Work out the finished part from the listing and answer in its coordinate system (mm). Face numbers are marked on the shaded views. A direction names the side the tool comes from. Give positions to 0.01 mm unless a question says otherwise; leave off trailing zeros. Loops run counter-clockwise (first coordinate to the right, second up) from the corner with the lowest first, then second, coordinate; pieces in that order, holes last. Notation, with made-up numbers: (-39, -4) - (-4, -4) arc R16 cw to (-4, 13) - close; hole circle Ø3 at (61, -2). An arc over 180 degrees is marked (long way). One line per item, written item: value.
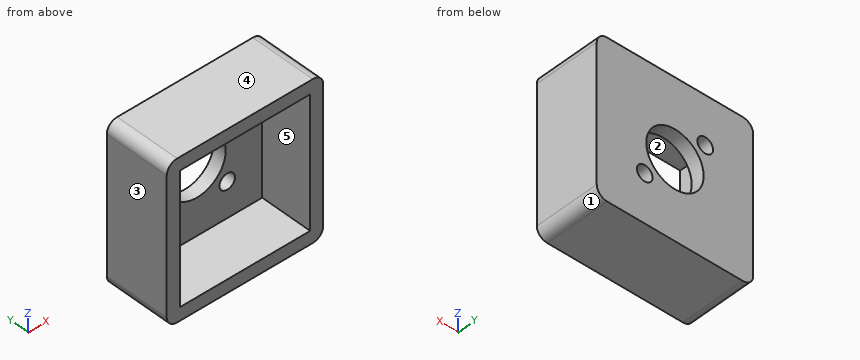
from build123d import *

# Parameters (mm, degrees)
SKETCH1_W           = 38.1
SKETCH1_H           = 38.1
SKETCH1_R           = 1.905
SKETCH1_R_2         = 6.985
BOSS_EXTRUDE1_DEPTH = 3.175
SKETCH1_3_W         = 38.1
SKETCH1_3_H         = 38.1
SKETCH1_3_W_2       = 31.75
SKETCH1_3_H_2       = 31.75
BOSS_EXTRUDE2_DEPTH = 12.7
FILLET1_R           = 2.54


with BuildPart() as part:
    # Sketch1 → Boss-Extrude1 (new body)
    with BuildSketch(Plane(origin=(0, 0, 0), x_dir=(1, 0, 0), z_dir=(0, 1, 0))):
        Rectangle(SKETCH1_W, SKETCH1_H)
        with Locations(Location((-7.363810019, -7.363810019, 0), (0, 0, 270))):
            Circle(SKETCH1_R, mode=Mode.SUBTRACT)
        with Locations(Location((7.363810019, 7.363810019, 0), (0, 0, 270))):
            Circle(SKETCH1_R, mode=Mode.SUBTRACT)
        with Locations(Location((0, 0, 0), (0, 0, 270))):
            Circle(SKETCH1_R_2, mode=Mode.SUBTRACT)
    extrude(amount=BOSS_EXTRUDE1_DEPTH)

    # Sketch1_3 → Boss-Extrude2 (add)
    with BuildSketch(Plane(origin=(0, 0, 0), x_dir=(1, 0, 0), z_dir=(0, 1, 0))):
        Rectangle(SKETCH1_3_W, SKETCH1_3_H)
        Rectangle(SKETCH1_3_W_2, SKETCH1_3_H_2, mode=Mode.SUBTRACT)
    extrude(amount=-BOSS_EXTRUDE2_DEPTH)

    # Fillet1
    fillet1_edges = [part.edges().sort_by_distance(p)[0] for p in [
        (-19.05, -4.7625, 19.05),
        (-19.05, -4.7625, -19.05),
        (19.05, -4.7625, -19.05),
        (19.05, -4.7625, 19.05),
    ]]
    fillet(fillet1_edges, radius=FILLET1_R)


solid = part.part
1. Section D-D (x = 12) is taken. Write down the section's boundary in (y, z) (3 decimals), and give its area (3 significant figures).
Output:
outline: (-12.7, -19.05) - (3.175, -19.05) - (3.175, 19.05) - (-12.7, 19.05) - (-12.7, 15.875) - (0, 15.875) - (0, -15.875) - (-12.7, -15.875) - close
area: 202 mm²
2. The mould has two halves that part along Z. Classify the marked faces 3, 4 and 5: released by +Z, released by -Z, zero draft, split by the parting line, or undercut.
Output:
face 3: zero draft
face 4: released by +Z
face 5: undercut
3. Find the intervals of material crossed by line 1 along Z through (x, y) = (6.5, -4) (3 decimals); line 2 along Y through (x, z) = (-5.5, 12) (3 decimals), in increasing order.
Output:
line 1: z = -19.05 to -15.875, 15.875 to 19.05
line 2: y = 0 to 3.175
4. Section C-C (y = -3.75) is taken. Write down the section's boundary in (x, z) (3 decimals).
Output:
outline: (-19.05, -16.51) arc R2.54 ccw to (-16.51, -19.05) - (16.51, -19.05) arc R2.54 ccw to (19.05, -16.51) - (19.05, 16.51) arc R2.54 ccw to (16.51, 19.05) - (-16.51, 19.05) arc R2.54 ccw to (-19.05, 16.51) - close; hole (-15.875, -15.875) - (15.875, -15.875) - (15.875, 15.875) - (-15.875, 15.875) - close
5. Flat-ended cylindrical pins translate along their axes: pin 1 Ø1 at (x, z) = (10, -0.5) entering from -Y; pin 2 Ø4.5 at (x, z) = (-7.36, 7.36) entering from +Y (3 decimals). Find the tip coordinate at first contact, or state that the pin passes through.
Output:
pin 1: stops at y = 0
pin 2: stops at y = 3.175
6. Section B-B (z = 0) is taken. Write down the section's boundary in (x, y) (3 decimals).
Output:
outline: (-19.05, -12.7) - (-15.875, -12.7) - (-15.875, 0) - (-6.985, 0) - (-6.985, 3.175) - (-19.05, 3.175) - close; (6.985, 0) - (15.875, 0) - (15.875, -12.7) - (19.05, -12.7) - (19.05, 3.175) - (6.985, 3.175) - close
7. For the marked faces 1 and 2, determine the directions among +Z, -Z, +X, -X, +Y, -Y from which every point of the face is accessible in a straight line to the end or side of a thin tool.
Output:
face 1: -Z, +X, +Y, -Y
face 2: -Y
8. Section A-A (x = 0) is taken. Write down the section's boundary in (y, z) (3 decimals), and give its area (3 significant figures).
Output:
outline: (-12.7, -19.05) - (3.175, -19.05) - (3.175, -6.985) - (0, -6.985) - (0, -15.875) - (-12.7, -15.875) - close; (-12.7, 15.875) - (0, 15.875) - (0, 6.985) - (3.175, 6.985) - (3.175, 19.05) - (-12.7, 19.05) - close
area: 157 mm²
